Work out the finished part from the listing and answer in its coordinate system (mm). Round coordinates to 2 decimals unless told otherwise and drop trailing zeros. Write each loop counter-clockwise with the first axis right and the second up, starting at its lowest first coordinate (ties: lowest second). Pieces come first, ordered by that corner, then holes.
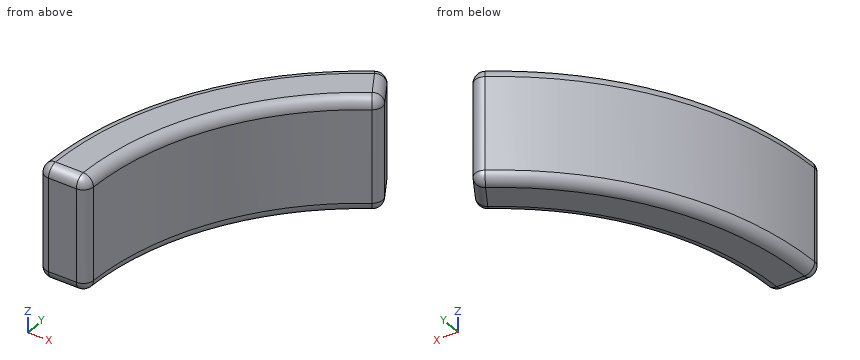
from build123d import *

# Parameters (mm, degrees)
BOSS_EXTRUDE1_DEPTH = 331.6
FILLET1_R           = 30


with BuildPart() as part:
    # Sketch1 → Boss-Extrude1 (new body)
    with BuildSketch(Plane.XY):
        with BuildLine():
            Line((-791.6, 0), (-931.6, 0))
            ThreePointArc((-931.6, 0), (-806.789266166, 465.8), (-465.8, 806.789266166))
            Line((-465.8, 806.789266166), (-395.8, 685.545709636))
            ThreePointArc((-395.8, 685.545709636), (-685.545709636, 395.8), (-791.6, 0))
        make_face()
    extrude(amount=-BOSS_EXTRUDE1_DEPTH)

    # Fillet1
    fillet1_edges = [part.edges().sort_by_distance(p)[0] for p in [
        (-806.789266166, 465.8, -331.6),
        (-861.6, 0, -331.6),
        (-685.545709636, 395.8, -331.6),
        (-861.6, 0, 0),
        (-806.789266166, 465.8, 0),
        (-430.8, 746.167487901, 0),
        (-685.545709636, 395.8, 0),
        (-791.6, 0, -165.8),
        (-931.6, 0, -165.8),
        (-465.8, 806.789266166, -165.8),
        (-395.8, 685.545709636, -165.8),
        (-430.8, 746.167487901, -331.6),
    ]]
    fillet(fillet1_edges, radius=FILLET1_R)


solid = part.part
Q1. Find the intervals of material crossed by L1, parallel to X at y = 610.5, z = -175.5; L2, parallel to Y at x = -724.5, z = -212; L3, parallel to X at y = 365, z = -318, in increasing order.
Q2. Find section A-A (z = -127). Determine the outline of the cut face in (x, y).
Q3. Given pin 1 (12 mm diameter, centred on y = 676, z = -175, fed in from -X); pin 2 (1 mm diameter, centred on x = -592, z = -53.5, fed in from +Y); pin 3 (6 mm diameter, centred on y = 399.5, z = -81.5, fed in from -X), each flat-ended and moving along its own axis, determine where each tip first touches the part or whether it passes through.
Report:
1. L1: x = -703.68 to -503.91
1. L2: y = 318.95 to 585.64
1. L3: x = -851.81 to -707.92
2. outline: (-931.08, 31) arc R30 ccw to (-901.1, 0) - (-821.05, 0) arc R30 ccw to (-791.07, 28.9) arc R791.6 cw to (-420.57, 670.64) arc R30 ccw to (-410.53, 711.05) - (-450.55, 780.38) arc R30 ccw to (-492.39, 790.84) arc R931.6 ccw to start
3. pin 1: stops at x = -647.29
3. pin 2: stops at y = 719.73
3. pin 3: stops at x = -843.01
